Check sheet for the drawn part. Datum: minimum x, y, z corner. Units: mm. A direction names the side the tool comes from. Give positions to 0.01 mm unless a question says otherwise; leave off trailing zeros. Write each loop counter-clockwise with the first axis right and the second up, starting at its lowest first coordinate (ties: lowest second). Pieces come first, ordered by that corner, then holes. Notation, with made-up numbers: (88.25, 84) - (102.25, 84) arc R21 ccw to (102.25, 107) - close; hole circle Ø4 at (-34.75, -39.75). An arc over 180 degrees is marked (long way). Answer as a JSON object with one key per item and string values. Group by question number.
Item 1: Tool access check on the marked faces 1 and 2. Record the directions out of +Z, -Z, +X, -X, +Y, -Y that give a thin tool (end or side, any length) a straight path to the whole face; none if there is none.
Item 2: Scan lines: line 1 along X through (y, z) = (45, 22) (3 decimals); line 2 along Z through (x, y) = (17, 43) (3 decimals). Record each from-to range of solid material in increasing order. Write a range as [from, to].
Item 3: Sectioned sample at B-B, the plane x = 12.5. Record the boundary of the cut face in (y, z) (3 decimals).
Item 4: Draft check along Z on the marked faces 3, 4 and 5. Enter one of: +Z half, -Z half, draft (parallel to the pull), parting line (faces both ways), or undercut.
Item 5: Sectioned sample at C-C, the plane y = 111. Record the boundary of the cut face in (x, z) (3 decimals).
Item 6: Sectioned sample at A-A, the plane z = 19. Record the boundary of the cut face in (x, y) (3 decimals).
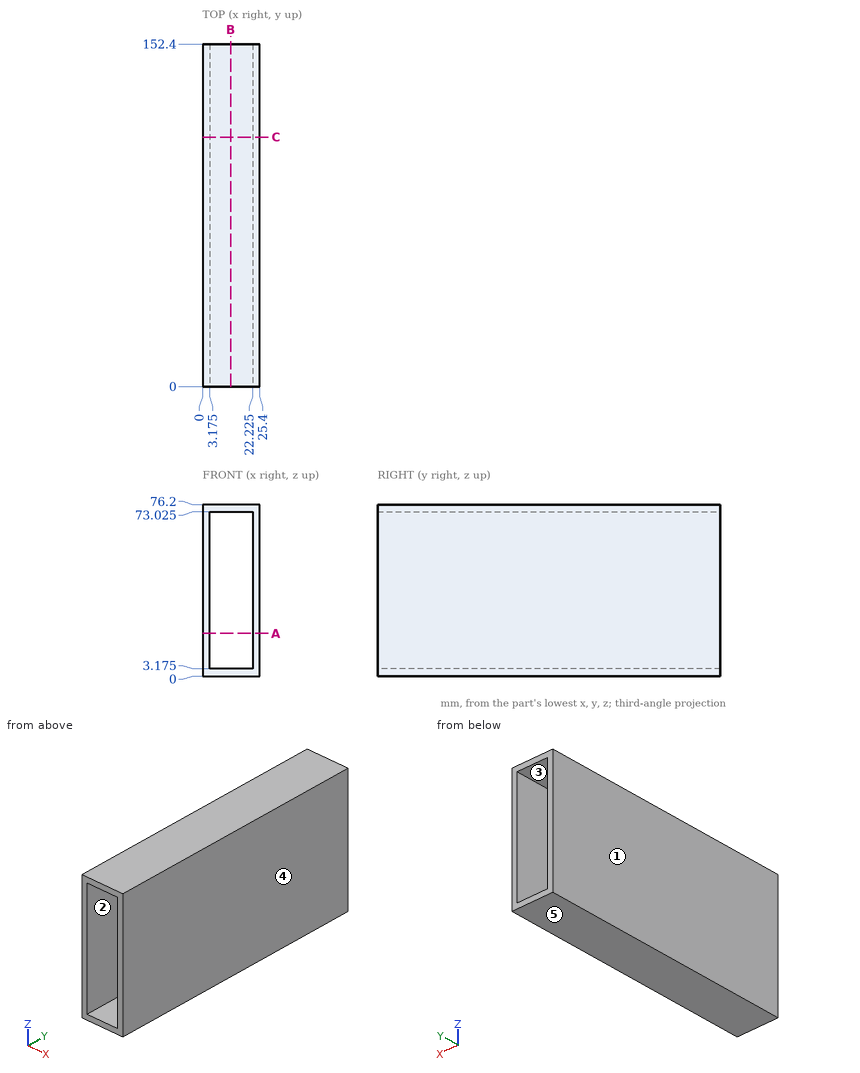
Geometry check:
{
 "1": {"face 1": "+Z, -Z, -X, +Y, -Y", "face 2": "+Y, -Y"},
 "2": {"line 1": "[0, 3.175], [22.225, 25.4]", "line 2": "[0, 3.175], [73.025, 76.2]"},
 "3": {"outline": "(0, 0) - (152.4, 0) - (152.4, 3.175) - (0, 3.175) - close; (0, 73.025) - (152.4, 73.025) - (152.4, 76.2) - (0, 76.2) - close"},
 "4": {"face 3": "undercut", "face 4": "draft", "face 5": "-Z half"},
 "5": {"outline": "(0, 0) - (25.4, 0) - (25.4, 76.2) - (0, 76.2) - close; hole (3.175, 3.175) - (22.225, 3.175) - (22.225, 73.025) - (3.175, 73.025) - close"},
 "6": {"outline": "(0, 0) - (3.175, 0) - (3.175, 152.4) - (0, 152.4) - close; (22.225, 0) - (25.4, 0) - (25.4, 152.4) - (22.225, 152.4) - close"}
}
